from build123d import *

# Parameters (mm, degrees)
F0_W     = 34.925
F0_H     = 34.925
F1_DEPTH = 2.54
F2_R     = 6.35
F3_DEPTH = 2.54


with BuildPart() as f1:
    # F0 (on Top) → F1 (new body)
    with BuildSketch(Plane.XY):
        with Locations((-17.4625, 17.4625)):
            Rectangle(F0_W, F0_H)
    extrude(amount=F1_DEPTH)

    # F2 (on face) → F3 (join)
    with BuildSketch(Plane(origin=(0, 0, 0), x_dir=(1, 0, 0), z_dir=(0, 0, -1))):
        with Locations((-17.4625, -17.4625)):
            Circle(F2_R)
    extrude(amount=F3_DEPTH)


solid = f1.part
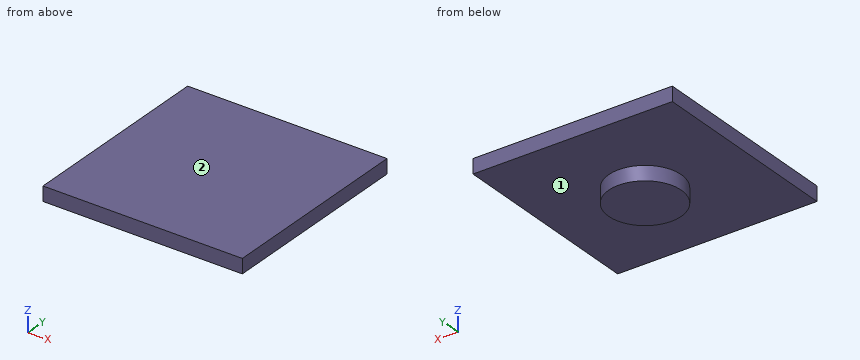
Can you work these out from the model? Positions are in its coordinate system, mm. Face numbers are marked on the shaded views. A direction names the side the tool comes from. Round coordinates to 2 decimals unless told otherwise and drop trailing zeros. Order: outer loops, then holes, each group sorted by start corner. A loop starts at its lowest first (then second) coordinate and runs counter-clockwise, first axis right, second up. Notation, with made-up numbers: M 37,51.25 L 70,51.25 A18 cw 70,70.25 Z; hole C -36,-19.5 d9. An arc over 180 degrees is marked long. Use a Markdown table: item, result.
1) On a 3-axis mill with a long thin cutter (end or side, diameter ignored), from which of +Z, -Z, +X, -X, +Y, -Y can I reach the whole of each face in a straight line? I mean the marked faces 1 and 2. Say none if no direction works.
Geometry says:
| item | result |
|---|---|
| face 1 | -Z |
| face 2 | +Z, +X, -X, +Y, -Y |
2) Imagine slicing it at C-C (z = -0.5). List the corners of the cut face in (x, y) for me.
Geometry says:
| item | result |
|---|---|
| outline | C -17.46,17.46 d12.7 |
3) Imagine slicing it at A-A (y = 32). List the corners of the cut face in (x, z) for me (3 decimals), then the cut area to 3 significant figures.
Geometry says:
| item | result |
|---|---|
| outline | M -34.925,0 L 0,0 L 0,2.54 L -34.925,2.54 Z |
| area | 88.7 mm² |
4) Imagine slicing it at D-D (y = 16.5). List the corners of the cut face in (x, z) for me (3 decimals).
Geometry says:
| item | result |
|---|---|
| outline | M -34.925,0 L -23.739,0 L -23.739,-2.54 L -11.186,-2.54 L -11.186,0 L 0,0 L 0,2.54 L -34.925,2.54 Z |
5) I'm going to push flat-ended pins straight in: P1, Ø1, axis at x = -28, z = -1.5, coming from the +Y side; P2, Ø5, axis at x = -28.5, y = 29.5, coming from the -Z side. Where does each tip first touch, or does it pass through?
Geometry says:
| item | result |
|---|---|
| P1 | passes through |
| P2 | stops at z = 0 |
6) Imagine slicing it at B-B (x = -7). List the corners of the cut face in (y, z) for me (3 decimals), then the cut area to 3 significant figures.
Geometry says:
| item | result |
|---|---|
| outline | M 0,0 L 34.925,0 L 34.925,2.54 L 0,2.54 Z |
| area | 88.7 mm² |
7) If I drill on line 1 along Z through (x, y) = (-4, 12.5); line 2 along Y through (x, z) = (-18, -1.65); line 3 along Y through (x, z) = (-13.5, -0.05), over which ranges is the centre line in solid material (lowest first)?
Geometry says:
| item | result |
|---|---|
| line 1 | z = 0 to 2.54 |
| line 2 | y = 11.14 to 23.79 |
| line 3 | y = 12.5 to 22.42 |
